The listing builds one solid part. Answer for the finished solid, in the listing's coordinates (mm). A direction names the side the tool comes from. Round coordinates to 2 decimals unless told otherwise and drop trailing zeros. Write each loop counter-clockwise with the first axis right and the second up, starting at its lowest first coordinate (ties: lowest second). Pieces come first, ordered by that corner, then holes.
from build123d import *

# Parameters (mm, degrees)
SKETCH020_W             = 40
SKETCH020_H             = 27
SKETCH020_R             = 1.9
PAD007_DEPTH            = 3
SKETCH021_W             = 3
SKETCH021_H             = 6
PAD008_DEPTH            = 3
SKETCH021_MIRRORED_2_W  = 3
SKETCH021_MIRRORED_2_H  = 6
PAD008_MIRRORED_2_DEPTH = 3
POCKET013_DEPTH         = 109.846683
BODY005_ROLL_ANGLE      = -90
BODY005_PLACEMENT_ANGLE = -10


with BuildPart() as part:
    # Sketch020 → Pad007 (new body)
    with BuildSketch(Plane.YZ):
        Rectangle(SKETCH020_W, SKETCH020_H)
        with Locations((0, 8.5)):
            Circle(SKETCH020_R, mode=Mode.SUBTRACT)
    extrude(amount=PAD007_DEPTH)

    # Sketch021 (on Face7 of Pad007) → Pad008 (join)
    with BuildSketch(Plane.YZ.offset(3)):
        with Locations((-21.5, 10.5)):
            Rectangle(SKETCH021_W, SKETCH021_H)
    pad008 = extrude(amount=-PAD008_DEPTH)

    # Sketch021 Mirrored 2 → Pad008 Mirrored 2 (add)
    with BuildSketch(Plane(origin=(3, 0, 0), x_dir=(0, -1, 0), z_dir=(-1, 0, 0))):
        with Locations((-21.5, 10.5)):
            Rectangle(SKETCH021_MIRRORED_2_W, SKETCH021_MIRRORED_2_H)
    pad008_mirrored_2 = extrude(amount=PAD008_MIRRORED_2_DEPTH)

    # Mirrored001: Pad008, Pad008 Mirrored 2 across Sketch021 H_Axis
    add(pad008.mirror(Plane(origin=(3, 0, 0), x_dir=(1, 0, 0), z_dir=(0, 0, 1))))
    add(pad008_mirrored_2.mirror(Plane(origin=(3, 0, 0), x_dir=(1, 0, 0), z_dir=(0, 0, 1))))

    # Sketch022 (on Face12 of MultiTransform) → Pocket013 (cut, through all)
    with BuildSketch(Plane.YZ.offset(3)):
        Polygon((-20, 1.6), (-16, 1.6), (-16, 2.75), (-13.5, 2.75), (-13.5, 1.6), (-10, 1.6), (-10, -1.6), (-13.5, -1.6), (-13.5, -2.75), (-16, -2.75), (-16, -1.6), (-20, -1.6), align=None)
    pocket013 = extrude(amount=-POCKET013_DEPTH, mode=Mode.SUBTRACT)

    # Mirrored002: Pocket013 across Sketch022 V_Axis
    add(pocket013.mirror(Plane(origin=(3, 0, 0), x_dir=(1, 0, 0), z_dir=(0, 1, 0))), mode=Mode.SUBTRACT)


with BuildPart() as part_1:
    # Body005 roll: moved
    add(part.part.rotate(Axis((0, 0, 0), (1, 0, 0)), BODY005_ROLL_ANGLE))


with BuildPart() as part_2:
    # Body005 placement: moved
    add(part_1.part.moved(Location((-14.721708, -14.689711, -20))).rotate(Axis((-14.721708, -14.689711, -20), (0, 0, 1)), BODY005_PLACEMENT_ANGLE))


solid = part_2.part
1. For a pull along Z with two mould halves and no side action, classify faces 1 (the face through (-11, -5, 3)), 2 (the face through (-11.92, -7.57, -41.52)), 3 (the face through (-14, -17, -4)) as released by +Z, released by -Z, zero draft, split by the parting line, or undercut.
Geometry says:
face 1: released by +Z
face 2: zero draft
face 3: undercut
2. Straight lines are drawn through the part: line 1 along Z through (x, y) = (-10.5, -6.25); line 2 along Y through (x, z) = (-14.75, -6); line 3 along X through (y, z) = (-19.25, -32). For each, find the intervals that lie inside material, in ascending order.
Geometry says:
line 1: z = -43 to -21.82, -18.18 to 3
line 2: y = -28.39 to -17.48
line 3: x = -15.53 to -12.48
3. A tool of negligible diameter and unlimited length cuts with its end or side. For faces 4 (the face through (-13.5, -16.53, -8.27)), 5 (the face through (-13, -13, -33.5)), 6 (the face through (-14, -17, -6.5)), 7 (the face through (-12.946, -13.378, -38.028)), from which of +Z, -Z, +X, -X, +Y, -Y can it reach the whole face along a straight path? Write none if from no direction.
Geometry says:
face 4: +Z, +X
face 5: -X
face 6: +X
face 7: -Z, -X
4. Section D-D on y = -24.25 is taken. Determine the outline of the cut face in (x, z), plus the area to 3 significant figures.
Geometry says:
outline: (-16.41, -43) - (-13.36, -43) - (-13.36, 3) - (-16.41, 3) - close
area: 140 mm2
5. Section A-A on z = -34.5 is taken. Determine the outline of the cut face in (x, y), plus the area to 3 significant figures.
Geometry says:
outline: (-17.07, -27.98) - (-14.11, -28.51) - (-12.24, -17.92) - (-15.2, -17.4) - close; (-14.24, -11.98) - (-11.29, -12.5) - (-9.42, -1.92) - (-12.38, -1.39) - close
area: 64.5 mm2
6. Section B-B on z = -20.5 is taken. Determine the outline of the cut face in (x, y), plus the area to 3 significant figures.
Geometry says:
outline: (-17.07, -27.98) - (-14.11, -28.51) - (-10.61, -8.64) - (-13.56, -8.12) - close; (-12.93, -4.51) - (-9.97, -5.03) - (-9.42, -1.92) - (-12.38, -1.39) - close
area: 70.0 mm2
7. Section C-C on y = -19 is taken. Determine the outline of the cut face in (x, z), plus the area to 3 significant figures.
Geometry says:
outline: (-15.48, -40) - (-12.44, -40) - (-12.44, 0) - (-15.48, 0) - close
area: 122 mm2
8. Given pin 1 (4 mm diameter, centred on y = -5, z = -33.5, fed in from -X); pin 2 (4.5 mm diameter, centred on x = -11.5, y = -11.5, fed in from +Z); pin 3 (1.8 mm diameter, centred on x = -12.5, y = -12.5, fed in from -Z); pin 4 (4 mm diameter, centred on x = -14.5, z = -5, fed in from -Y), each flat-ended and moving along its own axis, determine where each tip first touches the part or whether it passes through.
Geometry says:
pin 1: stops at x = -13.37
pin 2: stops at z = 0
pin 3: stops at z = -40
pin 4: stops at y = -28.51
